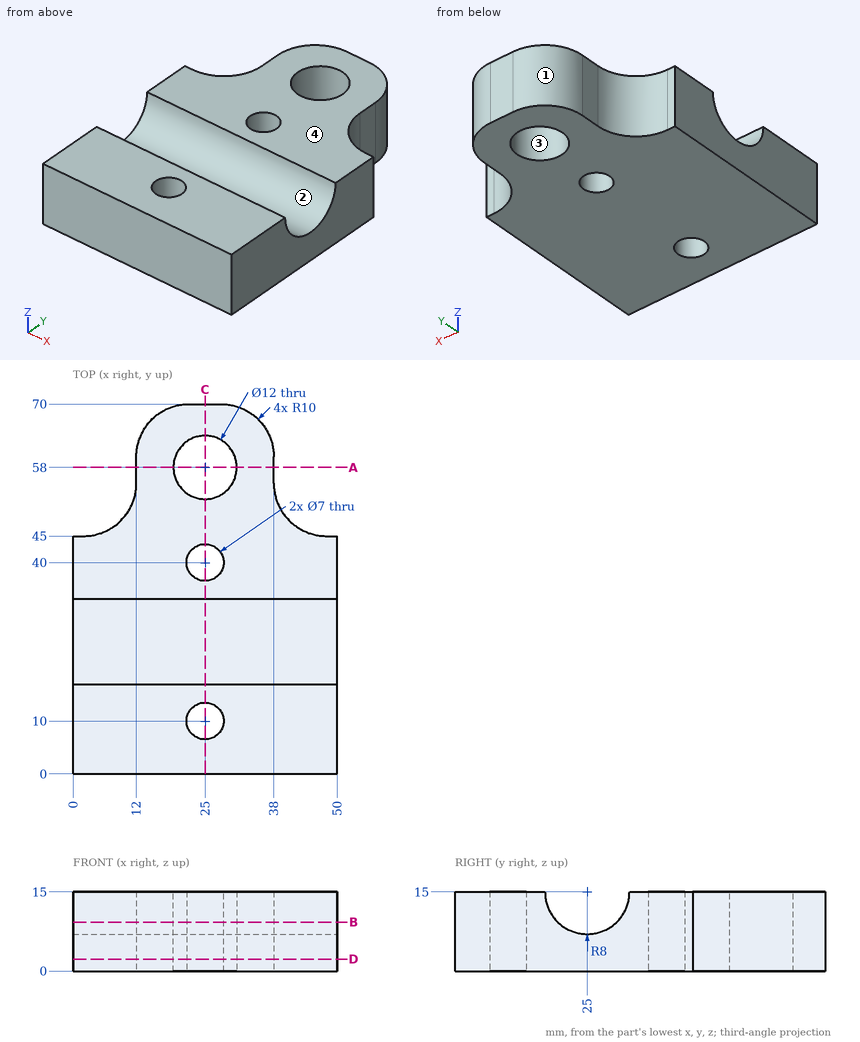
Design review of the part shown in the three views and the two pictorial views. Dimensions are in mm from the part's minimum x, y and z. Coordinates: 2 decimals unless noted, no trailing zeros. Order: outer loops, then holes, each group sorted by start corner. A loop starts at its lowest first (then second) coordinate and runs counter-clockwise, first axis right, second up.
1) Clearance check with flat-ended pins moving along their axes: pin 1 (8 mm diameter, centred on x = 6, z = 9.5, fed in from -Y); pin 2 (11 mm diameter, centred on x = 25, y = 58, fed in from -Z); pin 3 (1.6 mm diameter, centred on x = 1.5, z = 7, fed in from +Y); pin 4 (5.5 mm diameter, centred on y = 58.5, z = 11, fed in from +X). State where each tip first meets the part, or that it passes through.
2) Mouldability with a two-part tool opening along Y and no side actions: class the marked faces 1, 2, 3 and 4 as +Y half, -Y half, draft (parallel to the pull), parting line (faces both ways), or undercut.
3) Take a section at D-D, the plane z = 2.25. Give the boundary of the cut face in (x, y).
4) Wall thickness on line 1 along Y through (x, z) = (25, 5.75); line 2 along Y through (x, z) = (25, 11.5); line 3 along X through (y, z) = (10, 6.75): over which ranges is each line inside the solid? List them lowest first.
5) Take a section at B-B, the plane z = 9.25. Give the boundary of the cut face in (x, y), and give its area (3 significant figures).
6) Take a section at A-A, the plane y = 58. Give the boundary of the cut face in (x, z).
7) Take a section at C-C, the plane x = 25. Give the boundary of the cut face in (y, z).
Returned:
1. pin 1: stops at y = 0
1. pin 2: passes through
1. pin 3: stops at y = 45
1. pin 4: stops at x = 38
2. face 1: +Y half
2. face 2: undercut
2. face 3: undercut
2. face 4: draft
3. outline: (0, 0) - (50, 0) - (50, 45) - (48, 45) arc R10 cw to (38, 55) - (38, 60) arc R10 ccw to (28, 70) - (22, 70) arc R10 ccw to (12, 60) - (12, 55) arc R10 cw to (2, 45) - (0, 45) - close; hole circle Ø12 at (25, 58); hole circle Ø7 at (25, 10); hole circle Ø7 at (25, 40)
4. line 1: y = 0 to 6.5, 13.5 to 36.5, 43.5 to 52, 64 to 70
4. line 2: y = 0 to 6.5, 13.5 to 17.81, 32.19 to 36.5, 43.5 to 52, 64 to 70
4. line 3: x = 0 to 21.5, 28.5 to 50
5. outline: (0, 0) - (50, 0) - (50, 19.44) - (0, 19.44) - close; (0, 30.56) - (50, 30.56) - (50, 45) - (48, 45) arc R10 cw to (38, 55) - (38, 60) arc R10 ccw to (28, 70) - (22, 70) arc R10 ccw to (12, 60) - (12, 55) arc R10 cw to (2, 45) - (0, 45) - close; hole circle Ø12 at (25, 58); hole circle Ø7 at (25, 10); hole circle Ø7 at (25, 40)
5. area: 2,150 mm2
6. outline: (12, 0) - (19, 0) - (19, 15) - (12, 15) - close; (31, 0) - (38, 0) - (38, 15) - (31, 15) - close
7. outline: (0, 0) - (6.5, 0) - (6.5, 15) - (0, 15) - close; (13.5, 0) - (36.5, 0) - (36.5, 15) - (33, 15) arc R8 cw to (17, 15) - (13.5, 15) - close; (43.5, 0) - (52, 0) - (52, 15) - (43.5, 15) - close; (64, 0) - (70, 0) - (70, 15) - (64, 15) - close
